Check sheet for the modelled part. Datum: model origin and axes. Units: mm. A direction names the side the tool comes from. Coordinates: 2 decimals unless noted, no trailing zeros. Order: outer loops, then holes, each group sorted by start corner. A loop starts at its lowest first (then second) coordinate and runs counter-clockwise, first axis right, second up.
from build123d import *

# Parameters (mm, degrees)
F0_W     = 75
F0_H     = 35
F1_DEPTH = 5
F3_DEPTH = 25
F4_W     = 12
F4_H     = 12
F5_DEPTH = 39
F7_R     = 1.9
F8_DEPTH = 8
F9_R     = 2


with BuildPart() as f1:
    # F0 (on Top) → F1 (new body)
    with BuildSketch(Plane.XY):
        with Locations((37.5, 17.5)):
            Rectangle(F0_W, F0_H)
    extrude(amount=F1_DEPTH)

    # F2 (on face) → F3 (join)
    with BuildSketch(Plane.XZ):
        Polygon((25, 48.30127), (0, 5), (25, 5), align=None)
        Polygon((25, 48.30127), (25, 5), (50, 5), (50, 48.30127), (50, 118), (25, 118), align=None)
        Polygon((50, 48.30127), (50, 5), (75, 5), align=None)
    extrude(amount=-F3_DEPTH)

    # F4 (on face) → F5 (join)
    with BuildSketch(Plane.XY.offset(118)):
        with Locations((37.5, 12.5)):
            Rectangle(F4_W, F4_H)
    extrude(amount=F5_DEPTH)

    # F7 (on face) → F8 (cut)
    with BuildSketch(Plane(origin=(0, 0, 0), x_dir=(1, 0, 0), z_dir=(0, 0, -1))):
        with BuildLine():
            ThreePointArc((11.9, -15.5), (10, -13.6), (8.1, -15.5))
            Line((8.1, -15.5), (10, -15.5))
            Line((10, -15.5), (11.9, -15.5))
        make_face()
        with BuildLine():
            ThreePointArc((29.4, -15.5), (27.5, -13.6), (25.6, -15.5))
            ThreePointArc((25.6, -15.5), (27.5, -17.4), (29.4, -15.5))
        make_face()
        with BuildLine():
            Line((10, -15.5), (8.1, -15.5))
            ThreePointArc((8.1, -15.5), (10, -17.4), (11.9, -15.5))
            Line((11.9, -15.5), (10, -15.5))
        make_face()
        with Locations((47.5, -15.5)):
            Circle(F7_R)
        with Locations((65, -15.5)):
            Circle(F7_R)
    extrude(amount=-F8_DEPTH, mode=Mode.SUBTRACT)

    # F9
    f9_edges = [f1.edges().sort_by_distance(p)[0] for p in [
        (50, 0, 83.150635),
        (50, 25, 83.150635),
        (25, 25, 83.150635),
        (25, 0, 83.150635),
        (12.5, 0, 26.650635),
        (62.5, 0, 26.650635),
        (62.5, 25, 26.650635),
        (12.5, 25, 26.650635),
    ]]
    fillet(f9_edges, radius=F9_R)


solid = f1.part
(1) Go/stop test with flat-tipped pins: P1, Ø2, axis at y = 18.5, z = 21.5, coming from the -X side; P2, Ø3, axis at x = 47.5, y = 15.5, coming from the -Z side; P3, Ø13, axis at x = 38.5, z = 132, coming from the +Y side; P4, Ø5, axis at x = 10, y = 15.5, coming from the -Z side. Record where each tip stops, or that it passes through.
Filled in:
P1: stops at x = 8.95
P2: stops at z = 8
P3: stops at y = 18.5
P4: stops at z = 0
(2) Cross-section at B-B (x = 40.5). Enter the section's corners in (y, z).
Filled in:
outline: (0, 0) - (35, 0) - (35, 5) - (25, 5) - (25, 118) - (18.5, 118) - (18.5, 157) - (6.5, 157) - (6.5, 118) - (0, 118) - close
(3) Cross-section at D-D (y = 9). Enter the section's corners in (x, z).
Filled in:
outline: (0, 0) - (75, 0) - (75, 5) - (50, 48.3) - (50, 118) - (43.5, 118) - (43.5, 157) - (31.5, 157) - (31.5, 118) - (25, 118) - (25, 48.3) - (0, 5) - close
(4) Thickness scan on probe 1 along X at (y, z) = (15, 3); probe 2 along Y at (x, z) = (10, 2.25); probe 3 along X at (y, z) = (6.5, 58.5). Record the ranges inside material, lowest first.
Filled in:
probe 1: x = 0 to 8.17, 11.83 to 25.67, 29.33 to 45.67, 49.33 to 63.17, 66.83 to 75
probe 2: y = 0 to 13.6, 17.4 to 35
probe 3: x = 25 to 50
(5) Tool access check on faces 5 (the flat face through (25, 12, 84)), 6 (the flat face through (0, 17, 2)), 7 (the flat face through (43.5, 12, 137)), 8 (the cylindrical face through (49.312, 14.929, 3.944)). Record the directions out of +Z, -Z, +X, -X, +Y, -Y that give a thin tool (end or side, any length) a straight path to the whole face; none if there is none.
Filled in:
face 5: +Z, -X, +Y, -Y
face 6: +Z, -Z, -X, +Y, -Y
face 7: +Z, +X, +Y, -Y
face 8: -Z
(6) Cross-section at C-C (y = 15.5). Enter the section's corners in (x, z).
Filled in:
outline: (0, 0) - (8.1, 0) - (8.1, 8) - (11.9, 8) - (11.9, 0) - (25.6, 0) - (25.6, 8) - (29.4, 8) - (29.4, 0) - (45.6, 0) - (45.6, 8) - (49.4, 8) - (49.4, 0) - (63.1, 0) - (63.1, 8) - (66.9, 8) - (66.9, 0) - (75, 0) - (75, 5) - (50, 48.3) - (50, 118) - (43.5, 118) - (43.5, 157) - (31.5, 157) - (31.5, 118) - (25, 118) - (25, 48.3) - (0, 5) - close
(7) Cross-section at A-A (z = 106). Enter the section's corners in (x, y), and give its area (3 significant figures).
Filled in:
outline: (25, 2) arc R2 ccw to (27, 0) - (48, 0) arc R2 ccw to (50, 2) - (50, 23) arc R2 ccw to (48, 25) - (27, 25) arc R2 ccw to (25, 23) - close
area: 622 mm2
(8) Release check for a two-part mould opening along Y. For faces 1 (the flat face through (65, 15, 8)), 2 (the cylindrical face through (12.95, 24.4, 26.29)), 3 (the flat face through (31.5, 12, 137)), 4 (the flat face through (37, 6.5, 137)) record: +Y half, -Y half, draft (parallel to the pull), parting line (faces both ways), or undercut.
Filled in:
face 1: undercut
face 2: +Y half
face 3: draft
face 4: -Y half
